from build123d import *

# Parameters (mm, degrees)
F1_DEPTH = 10
F3_DEPTH = 5
F4_DEPTH = 5


with BuildPart() as f1:
    # F0 (on Top) → F1 (new body)
    with BuildSketch(Plane.XY):
        Polygon((44.978361, 74.922603), (-5.021639, 74.922603), (-50.021639, -75.077397), (-5.021639, -75.077397), (44.978361, -75.077397), (89.978361, -75.077397), align=None)
    extrude(amount=F1_DEPTH)

    # F2 (on face) → F3 (cut)
    with BuildSketch(Plane.XY.offset(10)):
        Polygon((44.978361, 74.922603), (39.758208, 74.922603), (84.758208, -75.077397), (89.978361, -75.077397), align=None)
        Polygon((-44.801485, -75.077397), (0.198515, 74.922603), (-5.021639, 74.922603), (-50.021639, -75.077397), align=None)
    extrude(amount=-F3_DEPTH, mode=Mode.SUBTRACT)

    # F2 (on face) → F4 (cut)
    with BuildSketch(Plane.XY.offset(10)):
        Polygon((44.978361, 74.922603), (39.758208, 74.922603), (84.758208, -75.077397), (89.978361, -75.077397), align=None)
        Polygon((-44.801485, -75.077397), (0.198515, 74.922603), (-5.021639, 74.922603), (-50.021639, -75.077397), align=None)
    extrude(amount=-F4_DEPTH, mode=Mode.SUBTRACT)


solid = f1.part
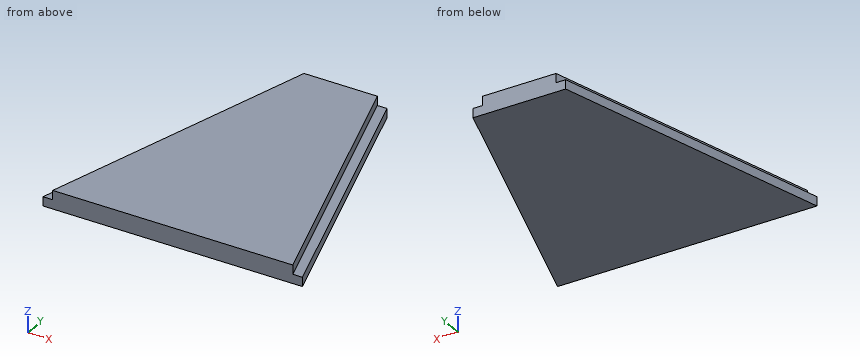
Design review of the part built by this model. Coordinates are the model's own, in mm. Coordinates: 2 decimals unless noted, no trailing zeros. Order: outer loops, then holes, each group sorted by start corner. A loop starts at its lowest first (then second) coordinate and runs counter-clockwise, first axis right, second up. Notation, with made-up numbers: (31, 18.5) -> (45, 18.5) arc R19 ccw to (45, 40.5) -> close; hole circle Ø3 at (62, 51). An arc over 180 degrees is marked (long way). Use one line per item in the form item = value. Start each with the question number.
(1) For probe 1 along Z at (x, y) = (60, 13.5); probe 2 along X at (y, z) = (-24, 9.5); probe 3 along X at (y, z) = (-63, 9.5), list the stretches that pass through material, from the lowest coordinate up.
(2) Add section B-B on x = 60. State the section outline as (y, z) points.
(3) Add section D-D on y = 20. State the section outline as (x, z) points, plus the area to 3 significant figures.
(4) Add section A-A on y = -7.5. State the section outline as (x, z) points, plus the area to 3 significant figures.
(5) Insertion check: pin 1 (10 mm diameter, centred on x = -19.5, y = 59, fed in from -Z); pin 2 (6 mm diameter, centred on y = 47, z = 2, fed in from +X). Each pin has a flat end and moves straight along its axis. Give the tip position at first contact, or say it passes through.
(6) Add section C-C on z = 1.5. State the section outline as (x, y) points, plus the area to 4 significant figures.
Answer block:
q1.probe_1 = 0 to 5
q1.probe_2 = -29.48 to 69.43
q1.probe_3 = -41.18 to 81.13
q2.outline = (-75.08, 0) -> (24.85, 0) -> (24.85, 5) -> (7.45, 5) -> (7.45, 10) -> (-75.08, 10) -> close
q3.outline = (-21.5, 0) -> (61.46, 0) -> (61.46, 5) -> (56.23, 5) -> (56.23, 10) -> (-16.28, 10) -> (-16.28, 5) -> (-21.5, 5) -> close
q3.area = 777 mm²
q4.outline = (-29.75, 0) -> (69.71, 0) -> (69.71, 5) -> (64.48, 5) -> (64.48, 10) -> (-24.53, 10) -> (-24.53, 5) -> (-29.75, 5) -> close
q4.area = 942 mm²
q5.pin_1 = through
q5.pin_2 = 54.26
q6.outline = (-50.02, -75.08) -> (89.98, -75.08) -> (44.98, 74.92) -> (-5.02, 74.92) -> close
q6.area = 14,250 mm²
